Answer from the drawing. Dimensions are ordinates in mm from the lowest x, y and z of the part. A direction names the side the tool comes from. Give positions to 0.01 mm unless a question says otherwise; leave off trailing zeros. Loops run counter-clockwise (first coordinate to the right, second up) from the corner with the lowest first, then second, coordinate; pieces in that order, holes last. Notation, with made-up numbers: (87, -34.5) - (116, -34.5) arc R26 ccw to (116, -20.5) - close; hole circle Ø11 at (16, 7). An arc over 180 degrees is marked (long way). Write each question's results on one line, items separated by ' | '. Start each with the question number.
Q1. For the marked faces 4, 5 and 6, determine the directions among +Z, -Z, +X, -X, +Y, -Y from which every point of the face is accessible in a straight line to the end or side of a thin tool.
Q2. Determine the mould class of the marked faces 1, 2 and 3 for opening direction X: +X half, -X half, draft (parallel to the pull), parting line (faces both ways), or undercut.
Q3. The part is cut by section D-D, the plane x = 6.5. Write down the section's boundary in (y, z).
Q4. Find the intervals of material crossed by line 1 (X direction, y = 56, z = 21.5); line 2 (X direction, y = 101, z = 22.5); line 3 (Z direction, x = 26, y = 92), in increasing order. Write a range as from..to.
Q5. Given pin 1 (8.5 mm diameter, centred on x = 24.5, y = 91, fed in from +Z), flat-ended and moving along its own axis, determine where the tip first touches the part or whether it passes through.
Q6. The part is cut by section B-B, the plane y = 56. Write down the section's boundary in (x, z).
Q7. The part is cut by section A-A, the plane z = 24. Write down the section's boundary in (x, y).
Q8. The part is cut by section C-C, the plane z = 38.5. Write down the section's boundary in (x, y), plus the area to 3 significant figures.
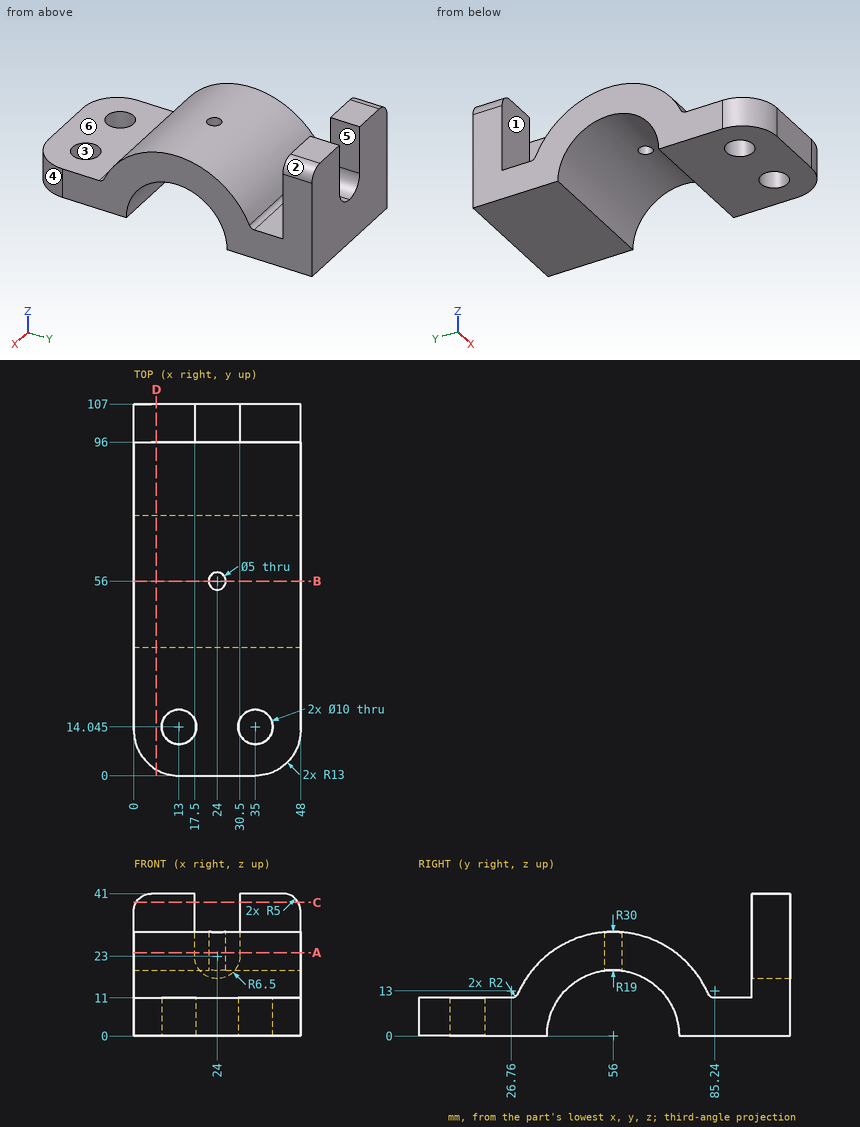
Check sheet entries:
1) face 4: +Z, -Z, +X, -Y | face 5: +Z, +Y | face 6: +Z, +X, -X, -Y
2) face 1: draft | face 2: +X half | face 3: undercut
3) outline: (1.74, 0) - (37, 0) arc R19 cw to (75, 0) - (107, 0) - (107, 41) - (96, 41) - (96, 11) - (85.24, 11) arc R2 cw to (83.41, 12.19) arc R30 ccw to (28.59, 12.19) arc R2 cw to (26.76, 11) - (1.74, 11) - close
4) line 1: x = 0..21.5, 26.5..48 | line 2: x = 0..17.52, 30.48..48 | line 3: z = 0..11
5) pin 1: stops at z = 11
6) outline: (0, 19) - (21.5, 19) - (21.5, 30) - (0, 30) - close; (26.5, 19) - (48, 19) - (48, 30) - (26.5, 30) - close
7) outline: (0, 38) - (48, 38) - (48, 74) - (0, 74) - close; (0, 96) - (17.5, 96) - (17.5, 107) - (0, 107) - close; (30.5, 96) - (48, 96) - (48, 107) - (30.5, 107) - close; hole circle Ø5 at (24, 56)
8) outline: (0.67, 96) - (17.5, 96) - (17.5, 107) - (0.67, 107) - close; (30.5, 96) - (47.33, 96) - (47.33, 107) - (30.5, 107) - close | area: 370 mm^2
